from build123d import *

# Parameters (mm, degrees)
SKETCH_1_W               = 65
SKETCH_1_H               = 15
EXTRUDE_1_DEPTH          = 2
SKETCH_2_R               = 1.25
SKETCH_2_R_2             = 3.45
SKETCH_2_R_3             = 1.5
SKETCH_2_R_4             = 1
CUT_EXTRUDE_1_DEPTH      = 2
SKETCH_4_R               = 1.5
EXTRUDE_2_DEPTH          = 2
SKETCH_5_R               = 7.5
SKETCH_5_R_2             = 7.2
EXTRUDE_3_DEPTH          = 6
SKETCH_5_8_R             = 1.25
SKETCH_5_8_R_2           = 7.2
EXTRUDE_4_DEPTH          = 6
CUT_EXTRUDE_2_DEPTH      = 3.5
CUT_EXTRUDE_2_DEPTH_BACK = 42.548164821
SKETCH_5_11_R            = 1.25
SKETCH_5_11_R_2          = 7.2
SKETCH_2_3_R             = 1.5
SKETCH_2_3_R_2           = 1
CUT_EXTRUDE_3_DEPTH      = 8


with BuildPart() as part:
    # 草图1 → 凸台-拉伸1 (new body)
    with BuildSketch(Plane(origin=(0, 0, 0), x_dir=(1, 0, 0), z_dir=(0, 1, 0))):
        with Locations((-7.5, 0)):
            Rectangle(SKETCH_1_W, SKETCH_1_H)
    extrude(amount=EXTRUDE_1_DEPTH)

    # 草图2 → 切除-拉伸1 (cut)
    with BuildSketch(Plane(origin=(0, 0, 0), x_dir=(1, 0, 0), z_dir=(0, 1, 0))):
        with Locations(Location((0, 0, 0), (0, 0, 270))):
            Circle(SKETCH_2_R)
        with Locations(Location((-16, 0, 0), (0, 0, 90))):
            Circle(SKETCH_2_R_2)
        with Locations(Location((-24, 0, 0), (0, 0, 90))):
            Circle(SKETCH_2_R)
        with Locations(Location((-32.5, 0, 0), (0, 0, 270))):
            Circle(SKETCH_2_R_3)
        with Locations(Location((-27, 0, 0), (0, 0, 270))):
            Circle(SKETCH_2_R_4)
        with Locations(Location((-32.5, -5.5, 0), (0, 0, 270))):
            Circle(SKETCH_2_R_4)
        with Locations(Location((-38, 0, 0), (0, 0, 270))):
            Circle(SKETCH_2_R_4)
        with Locations(Location((-32.5, 5.5, 0), (0, 0, 270))):
            Circle(SKETCH_2_R_4)
    extrude(amount=CUT_EXTRUDE_1_DEPTH, mode=Mode.SUBTRACT)

    # 草图4 → 凸台-拉伸2 (add)
    with BuildSketch(Plane.XY.offset(7.5)):
        with Locations(Location((20, 1, 0), (0, 0, 221.810314896))):
            Circle(SKETCH_4_R)
        with Locations(Location((-20, 1, 0), (0, 0, 221.810314896))):
            Circle(SKETCH_4_R)
    extrude(amount=EXTRUDE_2_DEPTH)

    # 草图5 → 凸台-拉伸3 (add)
    # profile 1 of 2: a face of its own
    with BuildSketch(Plane(origin=(0, 2, 0), x_dir=(1, 0, 0), z_dir=(0, 1, 0))):
        with Locations(Location((-32.5, 0, 0), (0, 0, 270))):
            Circle(SKETCH_5_R)
        with Locations(Location((-32.5, 0, 0), (0, 0, 270))):
            Circle(SKETCH_5_R_2, mode=Mode.SUBTRACT)
    # profile 2 of 2: a face of its own
    with BuildSketch(Plane(origin=(0, 2, 0), x_dir=(1, 0, 0), z_dir=(0, 1, 0))):
        with BuildLine():
            Line((5.149029035, -6.7), (-5.149029035, -6.7))
            ThreePointArc((-5.149029035, -6.7), (-8.45, 0), (-5.149029035, 6.7))
            Line((-5.149029035, 6.7), (5.149029035, 6.7))
            ThreePointArc((5.149029035, 6.7), (8.45, 0), (5.149029035, -6.7))
        make_face()
        with BuildLine():
            Line((4.905354218, -6), (-4.905354218, -6))
            ThreePointArc((-4.905354218, -6), (-7.75, 0), (-4.905354218, 6))
            Line((-4.905354218, 6), (4.905354218, 6))
            ThreePointArc((4.905354218, 6), (7.75, 0), (4.905354218, -6))
        make_face(mode=Mode.SUBTRACT)
    extrude(amount=EXTRUDE_3_DEPTH)

    # 草图5<8> → 凸台-拉伸4 (add)
    # profile 1 of 2: a face of its own
    with BuildSketch(Plane(origin=(0, 2, 0), x_dir=(1, 0, 0), z_dir=(0, 1, 0))):
        with BuildLine():
            Line((4.905354218, -6), (-4.905354218, -6))
            ThreePointArc((-4.905354218, -6), (-7.75, 0), (-4.905354218, 6))
            Line((-4.905354218, 6), (4.905354218, 6))
            ThreePointArc((4.905354218, 6), (7.75, 0), (4.905354218, -6))
        make_face()
        with Locations(Location((0, 0, 0), (0, 0, 270))):
            Circle(SKETCH_5_8_R, mode=Mode.SUBTRACT)
    # profile 2 of 2: a face of its own
    with BuildSketch(Plane(origin=(0, 2, 0), x_dir=(1, 0, 0), z_dir=(0, 1, 0))):
        with Locations((-32.5, 0)):
            Circle(SKETCH_5_8_R_2)
    extrude(amount=EXTRUDE_4_DEPTH)

    # 草图5<11> → 切除-拉伸2 (cut, two sides: drawn at the far end of the back side and taken through both)
    # profile 1 of 2: a face of its own
    with BuildSketch(Plane(origin=(0, 2, 0), x_dir=(1, 0, 0), z_dir=(0, 1, 0)).offset(-CUT_EXTRUDE_2_DEPTH_BACK)):
        with BuildLine():
            Line((4.905354218, -6), (-4.905354218, -6))
            ThreePointArc((-4.905354218, -6), (-7.75, 0), (-4.905354218, 6))
            Line((-4.905354218, 6), (4.905354218, 6))
            ThreePointArc((4.905354218, 6), (7.75, 0), (4.905354218, -6))
        make_face()
        with Locations(Location((0, 0, 0), (0, 0, 270))):
            Circle(SKETCH_5_11_R, mode=Mode.SUBTRACT)
    # profile 2 of 2: a face of its own
    with BuildSketch(Plane(origin=(0, 2, 0), x_dir=(1, 0, 0), z_dir=(0, 1, 0)).offset(-CUT_EXTRUDE_2_DEPTH_BACK)):
        with Locations(Location((-32.5, 0, 0), (0, 0, 270))):
            Circle(SKETCH_5_11_R_2)
    extrude(amount=CUT_EXTRUDE_2_DEPTH + CUT_EXTRUDE_2_DEPTH_BACK, mode=Mode.SUBTRACT)

    # 草图2<3> → 切除-拉伸3 (cut)
    with BuildSketch(Plane(origin=(0, 0, 0), x_dir=(1, 0, 0), z_dir=(0, 1, 0))):
        with Locations(Location((-32.5, 0, 0), (0, 0, 270))):
            Circle(SKETCH_2_3_R)
        with Locations(Location((-32.5, 5.5, 0), (0, 0, 270))):
            Circle(SKETCH_2_3_R_2)
        with Locations(Location((-38, 0, 0), (0, 0, 270))):
            Circle(SKETCH_2_3_R_2)
        with Locations(Location((-32.5, -5.5, 0), (0, 0, 270))):
            Circle(SKETCH_2_3_R_2)
        with Locations(Location((-27, 0, 0), (0, 0, 270))):
            Circle(SKETCH_2_3_R_2)
    extrude(amount=CUT_EXTRUDE_3_DEPTH, mode=Mode.SUBTRACT)


solid = part.part
Source: CAD feature listing. Evaluate the final solid. Frame: model axes, mm. A direction names the side the tool comes from. Round coordinates to 2 decimals unless told otherwise and drop trailing zeros. Loops run counter-clockwise (first coordinate to the right, second up) from the corner with the lowest first, then second, coordinate; pieces in that order, holes last. Notation, with made-up numbers: (-22, -39.5) -> (-13, -39.5) arc R22 ccw to (-13, -9.5) -> close; hole circle Ø8 at (14.25, 53.5). An arc over 180 degrees is marked (long way). Answer as a JSON object with one key per item and string values. Group by question number.
Q1. Section query A-A (y = 6.75). Output: boundary loops of the cut face in (x, z), plus the area to 3 significant figures.
Q2. Section query C-C (y = 1). Output: boundary loops of the cut face in (x, z).
Q3. Access query for faces 1 (the flat face through (-38, 2, -6)), 2 (the flat face through (-38, 2, 6)), 3 (the cylindrical face through (21.137, 0.022, 8.486)), 4 (the flat face through (-32, 5.5, -2)). Directions: +Z, -Z, +X, -X, +Y, -Y. A direction counts if a zero-diameter tool reaches every point of the face in a straight line with its end or side. Return the directions, or none.
Q4. Contact query for flat-ended pins moving along their axis: P1, Ø1, axis at x = 9, y = 1, coming from the +Z side; P2, Ø6, axis at x = 2.5, z = -2, coming from the -Y side; P3, Ø7.5, axis at x = -18, z = -1.5, coming from the +Y side. Output: stop coordinate, or through.
Q5. Section query B-B (x = -24). Output: boundary loops of the cut face in (y, z).
Q6. Section query D-D (x = 2). Output: boundary loops of the cut face in (y, z), plus the area to 3 significant figures.
Q7. Mould query, pull axis Z, two halves, no side actions, for faces 5 (the cylindrical face through (8.45, 4.96, -0.11)), 6 (the cylindrical face through (-19.42, 0.99, 0.45)), 7 (the flat face through (20, 1, 9.5)), 8 (the flat face through (0.1, 5.5, -1.4)). Classes: pulls with the +Z half, pulls with the -Z half, needs draft (parallel to the pull), parting line crosses it, or undercut.
Q8. Ray query, line 1 (X direction, y = 0.25, z = -4.75); line 2 (X direction, y = 3, z = 1.5); line 3 (X direction, y = 5.25, z = 3.75). Return the intervals inside material, ascending. Write a range as from..to.
Completed:
{
 "1": {"outline": "circle Ø15 at (-32.5, 0); (-5.15, -6.7) -> (5.15, -6.7) arc R8.45 ccw to (5.15, 6.7) -> (-5.15, 6.7) arc R8.45 ccw to start; hole circle Ø2 at (-38, 0); hole circle Ø3 at (-32.5, 0); hole circle Ø2 at (-32.5, -5.5); hole circle Ø2 at (-32.5, 5.5); hole circle Ø2 at (-27, 0); hole circle Ø2.5 at (0, 0)", "area": "352 mm²"},
 "2": {"outline": "(-40, -7.5) -> (25, -7.5) -> (25, 7.5) -> (21.5, 7.5) -> (21.5, 9.5) -> (18.5, 9.5) -> (18.5, 7.5) -> (-18.5, 7.5) -> (-18.5, 9.5) -> (-21.5, 9.5) -> (-21.5, 7.5) -> (-40, 7.5) -> close; hole circle Ø14.4 at (-32.5, 0); hole circle Ø2.5 at (-24, 0); hole circle Ø6.9 at (-16, 0); hole (-4.91, -6) -> (4.91, -6) arc R7.75 ccw to (4.91, 6) -> (-4.91, 6) arc R7.75 ccw to start"},
 "3": {"face 1": "-Z, -X, +Y", "face 2": "+Z, -X, +Y", "face 3": "+Z", "face 4": "-Y"},
 "4": {"P1": "z = 7.5", "P2": "y = 5.5", "P3": "y = 2"},
 "5": {"outline": "(0, -7.5) -> (2, -7.5) -> (2, -1.25) -> (0, -1.25) -> close; (0, 1.25) -> (2, 1.25) -> (2, 7.5) -> (0, 7.5) -> close"},
 "6": {"outline": "(0, -7.5) -> (2, -7.5) -> (2, -6.7) -> (8, -6.7) -> (8, 6.7) -> (2, 6.7) -> (2, 7.5) -> (0, 7.5) -> (0, 6) -> (5.5, 6) -> (5.5, -6) -> (0, -6) -> close", "area": "44.4 mm²"},
 "7": {"face 5": "parting line crosses it", "face 6": "undercut", "face 7": "pulls with the +Z half", "face 8": "undercut"},
 "8": {"line 1": "-40..-37.91, -27.09..-6.12, 6.12..25", "line 2": "-39.85..-39.54, -25.46..-25.15, -8.32..-7.6, 7.6..8.32", "line 3": "-39..-38.65, -26.35..-26, -7.57..-6.78, 6.78..7.57"}
}
